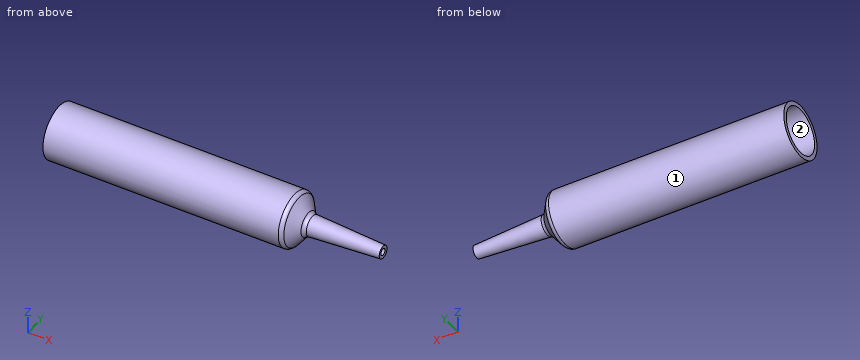
Autodesk Inventor part; units mm, degrees
ref_plane "YZ Plane" through (0, 0, 0) normal (1, 0, 0) x (0, 1, 0)
ref_plane "XZ Plane" through (0, 0, 0) normal (0, 1, 0) x (-1, 0, 0)
ref_plane "XY Plane" through (0, 0, 0) normal (0, 0, 1) x (1, 0, 0)
sketch "Skizze2" plane through (0, 0, 0) normal (0, 0, 1) x (1, 0, 0)
  line L0 (0, 0) -> (52.5603, 0) construction
  line L1 (0, 12.75) -> (0, 15)
  line L2 (0, 15) -> (131.1081, 15)
  line L3 (129.6756, 12.75) -> (0, 12.75)
  line L4 (0, 12.75) -> (0, 0) construction
  line L5 (180.3, 3.5) -> (140.9879, 5.6733)
  line L6 (138.7612, 6.8584) -> (133.5003, 13.8103)
  line L7 (180.3, 3.5) -> (180.2102, 1.875)
  line L8 (180.2102, 1.875) -> (139.0031, 4.153)
  line L9 (136.7765, 5.3381) -> (132.0678, 11.5603)
  arc A0 (133.5003, 13.8103) -> (131.1081, 15) centre (131.1081, 12) ccw
  arc A1 (138.7612, 6.8584) -> (140.9879, 5.6733) centre (141.1534, 8.6687) ccw
  arc A2 (132.0678, 11.5603) -> (129.6756, 12.75) centre (129.6756, 9.75) ccw
  arc A3 (136.7765, 5.3381) -> (139.0031, 4.153) centre (139.1687, 7.1485) ccw
  point P0 (132.6, 15)
  point P1 (131.1675, 12.75)
  point P2 (139.6, 5.75)
  point P3 (137.6153, 4.2298)
  dimension "d2" = 30
  dimension "d4" = 25.5
  dimension "d5" = 7
  dimension "d6" = 3.75
  dimension "d7" = 40.7
  dimension "d8" = 11.5
  dimension "d9" = 7
  dimension "d10" = 2.5
  dimension "d11" = 180.3
  dimension "d12" = 3
revolve "Umdrehung1" add sketch "Skizze2" angle 360 about axis through (0, 0, 0) along (1, 0, 0)
sketch "Skizze3" plane through (0, 0, 0) normal (-1, 0, 0) x (0, 0, 1)
  circle A0 centre (0, 0) radius 1.875
  arc A1 (0, 12.75) -> (-12.75, 0) centre (0, 0) ccw
  arc A2 (0, 16) -> (-5.7621, 14.9264) centre (0, 0) ccw
  line L0 (0, 0) -> (-25, 0)
  line L1 (-25, 0) -> (-25, 7.5)
  line L2 (-25, 7.5) -> (-5.7621, 14.9264)
  line L3 (0, 0) -> (0, 16)
  circle A3 centre (0, 0) radius 12.75
  dimension "d13" = 25
  dimension "d14" = 16
  dimension "d15" = 7.5
properties part number "P_Spritze_60ml" material "Glas"
The listing builds one solid part. Answer for the finished solid, in the listing's coordinates (mm). Face numbers are marked on the shaded views. Round coordinates to 2 decimals unless told otherwise and drop trailing zeros. Write each loop counter-clockwise with the first axis right and the second up, starting at its lowest first coordinate (ties: lowest second). Pieces come first, ordered by that corner, then holes. Notation, with made-up numbers: (46.25, -30) -> (56.25, -30) arc R28 ccw to (56.25, -9) -> close; hole circle Ø6 at (17, -40). An arc over 180 degrees is marked (long way). Write item = value, one per line.
1) For a pull along Z with two mould halves and no side action, classify the marked faces 1 and 2 as released by +Z, released by -Z, zero draft, split by the parting line, or undercut.
Check values:
face_1 = split by the parting line
face_2 = undercut
2) Straight lines are drawn through the part: line 1 along Z through (x, y) = (36, 0); line 2 along Z through (x, y) = (64, 11); line 3 along Y through (x, z) = (56, -7.25). For each, find the intervals that lie inside material, in ascending order. Write a range as [from, to].
Check values:
line_1 = [-15, -12.75], [12.75, 15]
line_2 = [-10.2, -6.45], [6.45, 10.2]
line_3 = [-13.13, -10.49], [10.49, 13.13]
3) Section D-D on x = 169.5 is taken. Write down the section's boundary in (y, z).
Check values:
outline = circle Ø8.19 at (0, 0); hole circle Ø4.93 at (0, 0)
4) Section C-C on x = 127.5 is taken. Write down the section's boundary in (y, z), plus the area to 3 significant figures.
Check values:
outline = circle Ø30 at (0, 0); hole circle Ø25.5 at (0, 0)
area = 196 mm²
5) Given pin 1 (5 mm diameter, centred on x = 119, z = 5.5, fed in from -Y); pin 2 (12 mm diameter, centred on y = -6, z = -11.5, fed in from +X); pin 3 (8 mm diameter, centred on x = 160, z = -2, fed in from -Y), each flat-ended and moving along its own axis, determine where each tip first touches the part or whether it passes through.
Check values:
pin_1 = -14.7
pin_2 = 138.68
pin_3 = -4.82
